```python
from build123d import *

# Parameters (mm, degrees)
CUT_EXTRUDE1_DEPTH      = 77.210235533
CUT_EXTRUDE1_DEPTH_BACK = 77.210235533
SKETCH3_W               = 43.997158999
SKETCH3_H               = 43.997158999
CUT_EXTRUDE2_DEPTH      = 76.916090791
SKETCH6_R               = 7.6
CUT_EXTRUDE3_DEPTH      = 77.203674452


with BuildPart() as part:
    # Sketch1 → Revolve1 (revolve)
    with BuildSketch(Plane.XY):
        with BuildLine():
            Line((0, 44), (0, -44))
            ThreePointArc((0, -44), (-44, 0), (0, 44))
        make_face()
    revolve(axis=Axis((0, 44, 0), (0, -1, 0)))

    # Sketch2 → Cut-Extrude1 (cut, two sides: drawn at the far end of the back side and taken through both)
    with BuildSketch(Plane(origin=(0, 0, 0), x_dir=(1, 0, 0), z_dir=(0, 1, 0)).offset(-CUT_EXTRUDE1_DEPTH_BACK)):
        with BuildLine():
            Line((-0.5, 43.997158999), (-0.5, 0.5))
            Line((-0.5, 0.5), (-43.997158999, 0.5))
            ThreePointArc((-43.997158999, 0.5), (31.112698372, -31.112698372), (-0.5, 43.997158999))
        make_face()
    extrude(amount=CUT_EXTRUDE1_DEPTH + CUT_EXTRUDE1_DEPTH_BACK, mode=Mode.SUBTRACT)

    # Sketch3 → Cut-Extrude2 (cut, through all)
    with BuildSketch(Plane(origin=(-0.5, 0, 0), x_dir=(0, 0, -1), z_dir=(1, 0, 0))):
        with Locations((21.998579499, -21.998579499)):
            Rectangle(SKETCH3_W, SKETCH3_H)
    extrude(amount=-CUT_EXTRUDE2_DEPTH, mode=Mode.SUBTRACT)

    # Sketch6 → Cut-Extrude3 (cut, through all)
    with BuildSketch(Plane.XZ):
        Circle(SKETCH6_R)
    extrude(amount=-CUT_EXTRUDE3_DEPTH, mode=Mode.SUBTRACT)


solid = part.part
```
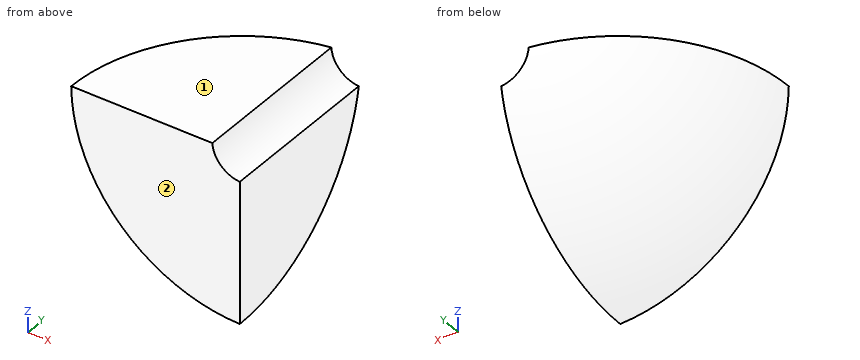
The model under review builds one solid part; all positions refer to its coordinate system, in mm. Face numbers are marked on the shaded views. Give positions to 0.01 mm unless a question says otherwise; leave off trailing zeros. Write each loop counter-clockwise with the first axis right and the second up, starting at its lowest first coordinate (ties: lowest second). Pieces come first, ordered by that corner, then holes. Notation, with made-up numbers: M 54,59.25 L 94,59.25 A26 cw 94,80.25 Z; hole C 13,-19 d11. An arc over 180 degrees is marked long. Write item = value, one per line. Start each with the question number.
Q1. We need section B-B (y = 29). State the section outline as (x, z) points.
Q2. We need section C-C (z = -12.5). State the section outline as (x, y) points, plus the area to 3 significant figures.
Q3. Mouldability with a two-part tool opening along Z and no side actions: class the marked faces 1 and 2 as released by +Z, released by -Z, zero draft, split by the parting line, or undercut.
Q4. Clearance check with flat-ended pins moving along their axes: pin 1 (3 mm diameter, centred on x = -35, y = 15.5, fed in from -Z); pin 2 (1.5 mm diameter, centred on x = -19, z = -36, fed in from +Y); pin 3 (4 mm diameter, centred on x = -19.5, y = 27.5, fed in from -Z). State where each tip first meets the part, or that it passes through.
Q5. For line 1 (X direction, y = 20, z = -36); line 2 (Z direction, x = -15.5, y = 38); line 3 (X direction, y = 32.5, z = -24), list the stretches that pass through material, from the lowest coordinate up.
Q6. We need section A-A (x = -15). State the section outline as (y, z) points, plus the area to 3 significant figures.
Q7. We need section D-D (y = 8). State the section outline as (x, z) points.
Result set:
q1.outline = M -33.09,-0.5 A33.09 ccw -0.5,-33.09 L -0.5,-7.58 A7.6 cw -7.58,-0.5 Z
q2.outline = M -42.19,0 L -0.5,0 L -0.5,42.18 A42.19 ccw Z
q2.area = 1,380 mm2
q3.face_1 = released by +Z
q3.face_2 = zero draft
q4.pin_1 = -24.15
q4.pin_2 = 18.43
q4.pin_3 = -30.5
q5.line_1 = -15.49 to -0.5
q5.line_2 = -15.87 to -0.5
q5.line_3 = -17.43 to -0.5
q6.outline = M 0,-41.36 A41.36 ccw 41.36,-0.5 L 0,-0.5 Z
q6.area = 1,320 mm2
q7.outline = M -43.26,-0.5 A43.27 ccw -0.5,-43.26 L -0.5,-7.58 A7.6 cw -7.58,-0.5 Z
